Check sheet for the modelled part. Datum: model origin and axes. Units: mm. Face numbers are marked on the shaded views. A direction names the side the tool comes from. Give positions to 0.01 mm unless a question says otherwise; leave off trailing zeros. Loops run counter-clockwise (first coordinate to the right, second up) from the corner with the lowest first, then second, coordinate; pieces in that order, holes last. Notation, with made-up numbers: (27, 10) -> (65, 10) arc R3 ccw to (65, 15) -> close; hole circle Ø8 at (79.25, 71.25). An arc over 180 degrees is marked (long way). Write each question's results on one line, items separated by ' | '. Start each with the question number.
1. Tool access check on the marked faces 1 and 2. Record the directions out of +Z, -Z, +X, -X, +Y, -Y that give a thin tool (end or side, any length) a straight path to the whole face; none if there is none.
2. Material ranges on L1, parallel to Z at x = 27.5, y = 0.55; L2, parallel to X at y = 28, z = -88, recorded low to high. Write a range as from..to.
3. Gauge pin test, flat ends, axial feed: pin 1 Ø12 at (y, z) = (29, -182.5) entering from +X; pin 2 Ø19 at (x, z) = (27.5, -212.5) entering from +Y. Record the tip position at first contact, or that the pin passes through.
4. Cross-section at C-C on z = -140.5. Record the boundary of the cut face in (x, y).
5. Cross-section at D-D on y = 38.5. Count the separate pieces of the cut face and the enclosed holes in it, and give its area (3 significant figures).
6. Cross-section at A-A on z = -112.5. Record the boundary of the cut face in (x, y).
7. Cross-section at B-B on x = 27.5. Record the boundary of the cut face in (y, z).
Autodesk Inventor part; units mm, degrees
ref_plane "YZ Plane" through (0, 0, 0) normal (1, 0, 0) x (0, 1, 0)
ref_plane "XZ Plane" through (0, 0, 0) normal (0, 1, 0) x (-1, 0, 0)
ref_plane "XY Plane" through (0, 0, 0) normal (0, 0, 1) x (1, 0, 0)
sketch "Sketch2" plane through (0, 0, 0) normal (1, 0, 0) x (0, 1, 0)
  line L0 (0, 0) -> (50, 0)
  line L1 (50, 0) -> (50, -225)
  line L2 (50, -225) -> (0, -225)
  line L3 (0, -225) -> (0, 0)
  dimension "d0" = 50
  dimension "d1" = 225
extrude "Plate1" add sketch "Sketch2" along normal blind 1.5
sketch "Sketch3" plane through (0, 1.5, -225) normal (0, -1, 0) x (1, 0, 0)
  line L0 (0, 225) -> (0, 0)
  line L1 (0, 0) -> (25.4, 0)
  line L2 (25.4, 0) -> (25.4, 225)
  line L3 (25.4, 225) -> (0, 225)
edge flange "Flange1" height 25.4 angle 90 thickness 1.5 bend radius 1.5 thickness toward (0, -1, 0) relief tear relief width 1.5 relief depth 0.75 edges at (1.5, 0, -112.5) wall of the first edge with corners at (0, 1.5, 0) (0, 1.5, -225) (25.4, 1.5, -225) (25.4, 1.5, 0)
bend "Bend1"
corner "Corner1"
sketch "Sketch4" plane through (25.4, 1.5, 0) normal (0, 1, 0) x (1, 0, 0)
  line L0 (-25.4, 0) -> (24.6, 0)
  line L1 (-22.4, 0) -> (0, 0)
  line L2 (-25.4, 0) -> (24.6, 0) construction
  line L3 (0, 225) -> (-22.4, 225)
  line L4 (24.6, 0) -> (-22.4, 0)
  line L5 (-22.4, 0) -> (-22.4, 225)
  line L6 (-22.4, 225) -> (24.6, 225)
  line L7 (24.6, 225) -> (24.6, 0)
  dimension "d13" = 50
  dimension "d14" = 0
sheet face with bend "Face2" sketch "Sketch4" thickness 1.5 toward (0, -1, 0) bend radius 1.5
bend "Bend2"
sketch "Sketch5" plane through (0, 50, 0) normal (0, 0, 1) x (1, 0, 0)
  point P0 (0, -50)
sketch "Sketch6" plane through (3, 1.5, 0) normal (0, 1, 0) x (1, 0, 0)
  line L0 (47, 225) -> (47, 0)
  line L1 (0, 0) -> (47, 0)
  line L2 (47, 225) -> (24.5, 225)
  line L3 (24.5, 225) -> (24.5, 0)
  line L4 (24.5, 0) -> (47, 0)
  line L5 (47, 0) -> (47, 225)
  circle A0 centre (24.5, 112.5) radius 6
  line L6 (24.5, 112.5) -> (24.5, 12.5)
  line L7 (24.5, 112.5) -> (124.5, 112.5) construction
  line L8 (24.5, 112.5) -> (24.5, 212.5)
  line L9 (24.5, 112.5) -> (124.5, 112.5) construction
  circle A1 centre (24.5, 212.5) radius 6
  circle A2 centre (24.5, 12.5) radius 6
  point P0 (-3, 0)
  dimension "d20" = 22.5
  dimension "d21" = 12
  dimension "d22" = 100
  dimension "d23" = 90
  dimension "d24" = 100
  dimension "d25" = 90
  dimension "d26" = 12
  dimension "d27" = 12
hole "Hole1" at (27.5, 1.5, -12.5) at (27.5, 1.5, -112.5) at (27.5, 1.5, -212.5) direction (0, -1, 0) diameter 12 end through all
fillet "Corner Round1" radius 6.35 4 edges at (50, 0.75, 0) (50, 0.75, -225) (0.75, 50, -225) (0.75, 50, 0)
sketch "Sketch7" plane through (1.5, 0, 0) normal (1, 0, 0) x (0, 0, -1)
  arc A0 (6.35, 50) -> (0, 43.65) centre (6.35, 43.65) ccw
  circle A1 centre (112.5, 35) radius 6.95
  line L0 (112.5, 35) -> (87.5, 35)
  line L1 (87.5, 35) -> (62.5, 35)
  line L2 (62.5, 35) -> (37.5, 35)
  line L3 (37.5, 35) -> (12.5, 35)
  circle A2 centre (12.5, 35) radius 6.95
  circle A3 centre (37.5, 35) radius 6.95
  circle A4 centre (62.5, 35) radius 6.95
  circle A5 centre (87.5, 35) radius 6.95
  line L4 (112.5, 35) -> (137.5, 35)
  line L5 (137.5, 35) -> (162.5, 35)
  line L6 (162.5, 35) -> (187.5, 35)
  line L7 (187.5, 35) -> (212.5, 35)
  circle A6 centre (137.5, 35) radius 6.95
  circle A7 centre (162.5, 35) radius 6.95
  circle A8 centre (187.5, 35) radius 6.95
  circle A9 centre (212.5, 35) radius 6.95
  point P0 (0, 0)
  dimension "d38" = 13.9
  dimension "d43" = 25
  dimension "d44" = 25
  dimension "d45" = 25
  dimension "d46" = 25
  dimension "d47" = 13.9
  dimension "d48" = 13.9
  dimension "d49" = 13.9
  dimension "d50" = 13.9
  dimension "d51" = 25
  dimension "d52" = 25
  dimension "d53" = 25
  dimension "d54" = 180
  dimension "d55" = 25
  dimension "d56" = 13.9
  dimension "d57" = 13.9
  dimension "d58" = 13.9
  dimension "d59" = 13.9
hole "Hole2" at (1.5, 35, -12.5) at (1.5, 35, -37.5) at (1.5, 35, -62.5) at (1.5, 35, -87.5) at (1.5, 35, -112.5) at (1.5, 35, -137.5) at (1.5, 35, -162.5) at (1.5, 35, -187.5) at (1.5, 35, -212.5) direction (-1, 0, 0) diameter 13.9 end through all
equation "\"d2\" = Thickness"
equation "\"d3\" = BendReliefWidth"
equation "\"d4\" = BendReliefDepth"
equation "\"d5\" = MinimumRemnant"
equation "\"d6\" = TransitionRadius"
equation "\"d9\" = BendRadius"
equation "\"d10\" = CornerReliefSize"
equation "\"d11\" = GapSize"
equation "\"d12\" = JacobiRadiusSize"
equation "\"d15\" = BendRadius"
equation "\"d16\" = BendReliefWidth"
equation "\"d18\" = MinimumRemnant"
equation "\"d17\" = BendReliefDepth"
equation "\"d19\" = TransitionRadius"
equation "\"BendRadius\" = Thickness"
equation "\"BendReliefWidth\" = Thickness"
equation "\"BendReliefDepth\" = 0.5 * Thickness"
equation "\"CornerReliefSize\" = 4 * Thickness"
equation "\"MinimumRemnant\" = 2 * Thickness"
equation "\"TransitionRadius\" = BendRadius"
equation "\"JacobiRadiusSize\" = BendRadius"
equation "\"GapSize\" = Thickness"
properties part number "Mounting_bracket"
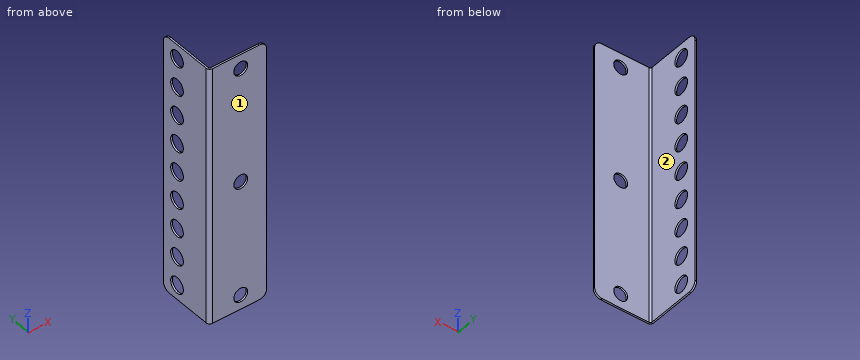
Geometry says:
1) face 1: +Z, -Z, +X, -X, -Y | face 2: +Z, -Z, +X, +Y
2) L1: -225..-218.5, -206.5..-118.5, -106.5..-18.5, -6.5..0 | L2: 0..1.5
3) pin 1: x = 1.5 | pin 2: y = 1.5
4) outline: (0, 3) arc R3 ccw to (3, 0) -> (50, 0) -> (50, 1.5) -> (3, 1.5) arc R1.5 cw to (1.5, 3) -> (1.5, 28.73) -> (0, 28.73) -> close; (0, 41.27) -> (1.5, 41.27) -> (1.5, 50) -> (0, 50) -> close
5) separate pieces: 10 | enclosed holes: 0 | area: 175 mm^2
6) outline: (0, 3) arc R3 ccw to (3, 0) -> (21.5, 0) -> (21.5, 1.5) -> (3, 1.5) arc R1.5 cw to (1.5, 3) -> (1.5, 28.05) -> (0, 28.05) -> close; (0, 41.95) -> (1.5, 41.95) -> (1.5, 50) -> (0, 50) -> close; (33.5, 0) -> (50, 0) -> (50, 1.5) -> (33.5, 1.5) -> close
7) outline: (0, -225) -> (1.5, -225) -> (1.5, -218.5) -> (0, -218.5) -> close; (0, -206.5) -> (1.5, -206.5) -> (1.5, -118.5) -> (0, -118.5) -> close; (0, -106.5) -> (1.5, -106.5) -> (1.5, -18.5) -> (0, -18.5) -> close; (0, -6.5) -> (1.5, -6.5) -> (1.5, 0) -> (0, 0) -> close
